The listing builds one solid part. Answer for the finished solid, in the listing's coordinates (mm). A direction names the side the tool comes from. Give positions to 0.01 mm unless a question says otherwise; leave off trailing zeros. Loops run counter-clockwise (first coordinate to the right, second up) from the corner with the lowest first, then second, coordinate; pieces in that order, holes last.
Item 1: Consider line 1 along Y through (x, z) = (0, 69); line 2 along Z through (x, y) = (0, -7.75); line 3 along Z through (x, y) = (-4.25, 7.25). Determine where each line is inside the solid, lowest interval first.
Item 2: Section D-D, the plane x = -6 is taken. Give the vertices of the cut face in (y, z).
Item 3: Section C-C, the plane z = 10 is taken. Give the vertices of the cut face in (x, y), and give its area (3 significant figures).
Item 4: The mould has two halves that part along Y. Classify faces 1 (the face through (0, 0, 70.2)), 2 (the face through (-1.02, -4.59, 69.34)), 3 (the face through (10, 3.2, 34.2)): pulls with the +Y half, pulls with the -Y half, needs draft (parallel to the pull), parting line crosses it, or undercut.
Item 5: Section A-A, the plane y = -6.75 is taken. Give the vertices of the cut face in (x, z), and give its area (3 significant figures).
Item 6: A tool of negligible diameter and unlimited length cuts with its end or side. For faces 4 (the face through (0, 0, 0)), 5 (the face through (3.44, -3.44, 68.5)), from which of +Z, -Z, +X, -X, +Y, -Y can it reach the whole face along a straight path? Write none if from no direction.
Item 7: Section B-B, the plane x = 1.5 is taken. Give the vertices of the cut face in (y, z), and give its area (3 significant figures).
Item 8: Each of these flat-tipped pins is pushed along its axis until it touches: pin 1 Ø2 at (x, y) = (-6, 4.5) entering from +Z; pin 2 Ø1 at (x, z) = (-1, 13) entering from -Y; pin 3 Ø1 at (x, z) = (2.5, 20) entering from -Y. Where does it stop, or does it pass through?
from build123d import *

# Parameters (mm, degrees)
SKETCH1_R           = 10.5
BOSS_EXTRUDE1_DEPTH = 68.50000016
SKETCH2_R           = 4.7
BOSS_EXTRUDE2_DEPTH = 1.7
SKETCH3_R           = 10.5
SKETCH3_R_2         = 8
BOSS_EXTRUDE3_DEPTH = 0.8


with BuildPart() as part:
    # Sketch1 → Boss-Extrude1 (new body)
    with BuildSketch(Plane.XY):
        Circle(SKETCH1_R)
    extrude(amount=BOSS_EXTRUDE1_DEPTH)

    # Sketch2 → Boss-Extrude2 (add)
    with BuildSketch(Plane.XY.offset(68.50000016)):
        Circle(SKETCH2_R)
    extrude(amount=BOSS_EXTRUDE2_DEPTH)

    # Sketch3 → Boss-Extrude3 (add)
    with BuildSketch(Plane.XY.offset(68.50000016)):
        Circle(SKETCH3_R)
        Circle(SKETCH3_R_2, mode=Mode.SUBTRACT)
    extrude(amount=BOSS_EXTRUDE3_DEPTH)


solid = part.part
Worked answers:
1. line 1: y = -10.5 to -8, -4.7 to 4.7, 8 to 10.5
1. line 2: z = 0 to 68.5
1. line 3: z = 0 to 69.3
2. outline: (-8.62, 0) - (8.62, 0) - (8.62, 69.3) - (5.29, 69.3) - (5.29, 68.5) - (-5.29, 68.5) - (-5.29, 69.3) - (-8.62, 69.3) - close
3. outline: circle Ø21 at (0, 0)
3. area: 346 mm2
4. face 1: needs draft
4. face 2: undercut
4. face 3: parting line crosses it
5. outline: (-8.04, 0) - (8.04, 0) - (8.04, 69.3) - (4.29, 69.3) - (4.29, 68.5) - (-4.29, 68.5) - (-4.29, 69.3) - (-8.04, 69.3) - close
5. area: 1,110 mm2
6. face 4: -Z, +X, -X, +Y, -Y
6. face 5: +Z
7. outline: (-10.39, 0) - (10.39, 0) - (10.39, 69.3) - (7.86, 69.3) - (7.86, 68.5) - (4.45, 68.5) - (4.45, 70.2) - (-4.45, 70.2) - (-4.45, 68.5) - (-7.86, 68.5) - (-7.86, 69.3) - (-10.39, 69.3) - close
7. area: 1,440 mm2
8. pin 1: stops at z = 69.3
8. pin 2: stops at y = -10.49
8. pin 3: stops at y = -10.31
